Source: CAD feature listing. Evaluate the final solid. Frame: model axes, mm. Face numbers are marked on the shaded views. Give positions to 0.01 mm unless a question says otherwise; leave off trailing zeros. Order: outer loops, then holes, each group sorted by start corner. A loop starts at its lowest first (then second) coordinate and runs counter-clockwise, first axis right, second up.
1) Section C-C, the plane y = 22. Return loops of the section in (x, z), plus the area to 3 significant figures.
2) First-contact query: P1, Ø1, axis at y = -31.5, z = 7, coming from the -X side; P2, Ø1.5, axis at y = -37, z = 9, coming from the -X side; P3, Ø4, axis at x = 57.5, z = 8.5, coming from the -Y side. Flat tips, straight axial feed; report the tip coordinate or a pass-through.
3) Material intervals for line 1 (Y direction, x = 0, z = 1); line 2 (X direction, y = -5, z = 1.9); line 3 (Z direction, x = 46, y = -13.5), sorted ascending.
4) Draft query along X for the marked faces 1 and 2. Return one class per face: released by +X, released by -X, zero draft, split by the parting line, or undercut.
5) Section A-A, the plane x = 17. Return loops of the section in (y, z).
6) Section B-B, the plane y = -51. Return loops of the section in (x, z).
```python
from build123d import *

# Parameters (mm, degrees)
BOSS_EXTRUDE1_DEPTH     = 3
BOSS_EXTRUDE2_DEPTH     = 6
FILLET1_R               = 20
FILLET2_R               = 6
FILLET4_R               = 3
SKETCH4_W               = 77.991272398
SKETCH4_H               = 3
BOSS_EXTRUDE3_DEPTH     = 8
FILLET5_R               = 3
CUT_EXTRUDE1_DEPTH      = 118
CUT_EXTRUDE1_DEPTH_BACK = 3
SKETCH5_R               = 1
SKETCH6_R               = 2
CUT_EXTRUDE2_DEPTH      = 6
FILLET6_R               = 3
SKETCH7_R               = 1
CUT_EXTRUDE3_DEPTH      = 3
SKETCH8_R               = 1
CUT_EXTRUDE4_DEPTH      = 3
SKETCH9_R               = 1
CUT_EXTRUDE5_DEPTH      = 3
SKETCH10_R              = 1
CUT_EXTRUDE6_DEPTH      = 3


with BuildPart() as part:
    # Sketch2 → Boss-Extrude1 (new body)
    with BuildSketch(Plane.XY):
        Polygon((85, 0), (85, 30), (-85, 30), (-85, 0), (-58.995636199, -70), (0, -80), (58.995636199, -70), align=None)
        Polygon((63.885527266, -33), (52.762165892, -62.942485887), (0, -71.885887347), (-52.762165892, -62.942485887), (-63.885527266, -33), align=None, mode=Mode.SUBTRACT)
    extrude(amount=BOSS_EXTRUDE1_DEPTH)

    # Sketch3 → Boss-Extrude2 (add)
    with BuildSketch(Plane.XY.offset(3)):
        Polygon((-74.691839611, -14.825881059), (-55.682056872, -65.99747679), (0, -75.435811633), (55.682056872, -65.99747679), (74.691839611, -14.825881059), (76.82538642, -14.825881059), (57.154758795, -67.776375994), (0, -77.464339796), (-57.154758795, -67.776375994), (-76.82538642, -14.825881059), align=None)
    extrude(amount=BOSS_EXTRUDE2_DEPTH)

    # Fillet1
    fillet1_edges = [part.edges().sort_by_distance(p)[0] for p in [
        (0, -71.885887347, 1.5),
        (0, -75.435811633, 6),
    ]]
    fillet(fillet1_edges, radius=FILLET1_R)

    # Fillet2
    fillet2_edges = [part.edges().sort_by_distance(p)[0] for p in [
        (-52.762165892, -62.942485887, 1.5),
        (52.762165892, -62.942485887, 1.5),
        (55.682056872, -65.99747679, 6),
        (-55.682056872, -65.99747679, 6),
    ]]
    fillet(fillet2_edges, radius=FILLET2_R)

    # Fillet4
    fillet4_edges = [part.edges().sort_by_distance(p)[0] for p in [
        (63.885527266, -33, 1.5),
        (-63.885527266, -33, 1.5),
    ]]
    fillet(fillet4_edges, radius=FILLET4_R)

    # Sketch4 → Boss-Extrude3 (add)
    with BuildSketch(Plane.XY.offset(3)):
        with Locations((0, -31.5)):
            Rectangle(SKETCH4_W, SKETCH4_H)
    extrude(amount=BOSS_EXTRUDE3_DEPTH)

    # Fillet5
    fillet5_edges = [part.edges().sort_by_distance(p)[0] for p in [
        (-38.995636199, -31.5, 3),
        (38.995636199, -31.5, 3),
        (-38.995636199, -31.5, 11),
        (38.995636199, -31.5, 11),
    ]]
    fillet(fillet5_edges, radius=FILLET5_R)

    # Sketch5 → Cut-Extrude1 (cut, two sides: drawn at the far end of the back side and taken through both)
    with BuildSketch(Plane.XY.offset(3).offset(-CUT_EXTRUDE1_DEPTH_BACK)):
        with Locations(Location((-65, 25, 0), (0, 0, 180))):
            Circle(SKETCH5_R)
        with Locations(Location((65, 25, 0), (0, 0, 180))):
            Circle(SKETCH5_R)
        with Locations(Location((0, 25, 0), (0, 0, 180))):
            Circle(SKETCH5_R)
        with Locations(Location((-77.808678419, -5, 0), (0, 0, 180))):
            Circle(SKETCH5_R)
        with Locations(Location((77.808678419, -5, 0), (0, 0, 180))):
            Circle(SKETCH5_R)
        with Locations(Location((-30, -69.84355772, 0), (0, 0, 200.379573945))):
            Circle(SKETCH5_R)
        with Locations(Location((30, -69.84355772, 0), (0, 0, 219.620426055))):
            Circle(SKETCH5_R)
    extrude(amount=CUT_EXTRUDE1_DEPTH + CUT_EXTRUDE1_DEPTH_BACK, mode=Mode.SUBTRACT)

    # Sketch6 → Cut-Extrude2 (cut)
    with BuildSketch(Plane.XY.offset(9)):
        with Locations((30, -69.84355772)):
            Circle(SKETCH6_R)
        with Locations((-30, -69.84355772)):
            Circle(SKETCH6_R)
    extrude(amount=-CUT_EXTRUDE2_DEPTH, mode=Mode.SUBTRACT)

    # Fillet6
    fillet6_edges = [part.edges().sort_by_distance(p)[0] for p in [
        (-75.758613015, -14.825881059, 9),
        (75.758613015, -14.825881059, 9),
    ]]
    fillet(fillet6_edges, radius=FILLET6_R)

    # Sketch7 → Cut-Extrude3 (cut)
    with BuildSketch(Plane(origin=(-72.348566579, -26.876834941, 0), x_dir=(0, 0, 1), z_dir=(-0.9374061965324084, -0.3482378823486089, 0))):
        with Locations(Location((6, 2.855637104, 0), (0, 0, 270))):
            Circle(SKETCH7_R)
        with Locations(Location((6, -33.630542667, 0), (0, 0, 270))):
            Circle(SKETCH7_R)
    extrude(amount=-CUT_EXTRUDE3_DEPTH, mode=Mode.SUBTRACT)

    # Sketch8 → Cut-Extrude4 (cut)
    with BuildSketch(Plane(origin=(72.348566579, -26.876834941, 0), x_dir=(0, 0, -1), z_dir=(0.9374061965324085, -0.3482378823486088, 0))):
        with Locations(Location((-6, 2.855637104, 0), (0, 0, 90))):
            Circle(SKETCH8_R)
        with Locations(Location((-6, -33.630542667, 0), (0, 0, 90))):
            Circle(SKETCH8_R)
    extrude(amount=-CUT_EXTRUDE4_DEPTH, mode=Mode.SUBTRACT)

    # Sketch9 → Cut-Extrude5 (cut)
    with BuildSketch(Plane(origin=(-12.429555178, -73.328951536, 0), x_dir=(0.9859365210363187, -0.1671202455922104, 0), z_dir=(0.1671202455922104, 0.9859365210363187, 0))):
        with Locations(Location((-1.969388477, -6, 0), (0, 0, 180))):
            Circle(SKETCH9_R)
        with Locations(Location((-30.024159445, -6, 0), (0, 0, 180))):
            Circle(SKETCH9_R)
    extrude(amount=-CUT_EXTRUDE5_DEPTH, mode=Mode.SUBTRACT)

    # Sketch10 → Cut-Extrude6 (cut)
    with BuildSketch(Plane(origin=(12.763795669, -75.300824578, 0), x_dir=(0.9859365210363187, 0.1671202455922103, 0), z_dir=(0.1671202455922103, -0.9859365210363187, 0))):
        with Locations((-0.945859491, 6)):
            Circle(SKETCH10_R)
        with Locations((33.024159445, 6)):
            Circle(SKETCH10_R)
    extrude(amount=-CUT_EXTRUDE6_DEPTH, mode=Mode.SUBTRACT)


solid = part.part
```
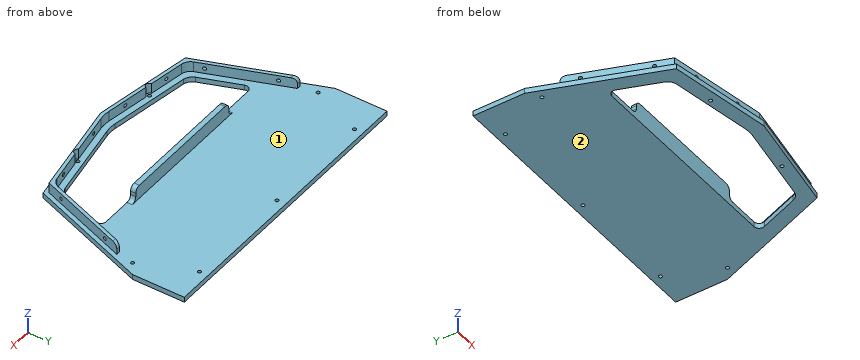
From the geometry:
1. outline: (-85, 0) - (85, 0) - (85, 3) - (-85, 3) - close
1. area: 510 mm2
2. P1: stops at x = -70.82
2. P2: stops at x = -68.87
2. P3: stops at y = -68.06
3. line 1: y = -80 to -71.6, -33 to 24, 26 to 30
3. line 2: x = -83.14 to -78.81, -76.81 to 76.81, 78.81 to 83.14
3. line 3: z = 0 to 3
4. face 1: undercut
4. face 2: zero draft
5. outline: (-77.12, 0) - (-69, 0) - (-69, 3) - (-72.55, 3) - (-72.55, 9) - (-74.58, 9) - (-74.58, 3) - (-77.12, 3) - close; (-33, 0) - (30, 0) - (30, 3) - (-30, 3) - (-30, 11) - (-33, 11) - close
6. outline: (-66.05, 0) - (-57.2, 0) - (-57.2, 3) - (-61.25, 3) - (-61.25, 9) - (-63.39, 9) - (-63.39, 3) - (-66.05, 3) - close; (57.2, 0) - (66.05, 0) - (66.05, 3) - (63.39, 3) - (63.39, 9) - (61.25, 9) - (61.25, 3) - (57.2, 3) - close
